Solid Edge part; units mm, degrees
sketch "Sketch1" plane through (0, 0, 0) normal (0, 0, 1) x (1, 0, 0)
  circle A0 centre (0, 0) radius 8.135
extrude "Protrusion1" add sketch "Sketch1" along normal blind 7
sketch "Sketch2" plane through (0, 0, 7) normal (0, 0, 1) x (1, 0, 0)
  line L0 (0, -2.8868) -> (-2.5, -1.4434)
  line L1 (-2.5, -1.4434) -> (-2.5, 1.4434)
  line L2 (-2.5, 1.4434) -> (0, 2.8868)
  line L3 (0, 2.8868) -> (2.5, 1.4434)
  line L4 (2.5, 1.4434) -> (2.5, -1.4434)
  line L5 (2.5, -1.4434) -> (0, -2.8868)
extrude "Cutout1" cut sketch "Sketch2" against normal blind 3.5
sketch "Sketch3" plane through (0, 0, 0) normal (0, 0, -1) x (0, 1, 0)
  circle A0 centre (0, 0) radius 5
extrude "Protrusion2" add sketch "Sketch3" along normal blind 40
sketch "Sketch4" plane through (0, 0, -40) normal (0, 0, -1) x (0, 1, 0)
  circle A0 centre (0, 0) radius 4
extrude "Protrusion3" add sketch "Sketch4" along normal blind 13
chamfer "Chamfer1" distance 0.5 angle 45 1 edges at (0, -4, -53)
properties part number "108082"
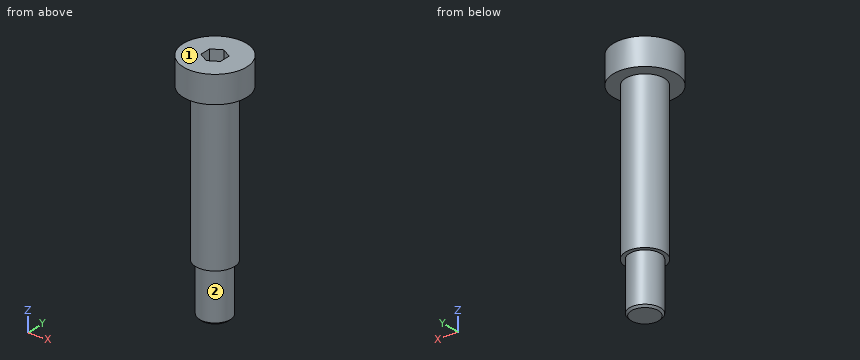
Could you check a few things on this model? Use its own coordinates, in mm. Face numbers are marked on the shaded views. A direction names the side the tool comes from. Round coordinates to 2 decimals unless told otherwise and drop trailing zeros. Loops run counter-clockwise (first coordinate to the right, second up) from the corner with the lowest first, then second, coordinate; pieces in that order, holes last. Notation, with made-up numbers: M 41,43.5 L 55,43.5 A12 cw 55,48.5 Z; hole C -17,27.25 d5. An arc over 180 degrees is marked long. Write item = value, one per line.
1. I want a section at D-D, the plane x = 6. Write out the boundary of the cut face in (y, z), and give its area (3 significant figures).
Results below:
outline = M -5.49,0 L 5.49,0 L 5.49,7 L -5.49,7 Z
area = 76.9 mm²
2. Which directions (+Z, -Z, +X, -X, +Y, -Y) give clear straight access to the entire face, cutting with the end or side of a thin tool? Please do the marked faces 1 and 2.
Results below:
face_1 = +Z, +X, -X, +Y, -Y
face_2 = -Z
3. I want a section at B-B, the plane z = -34. Write out the boundary of the cut face in (x, y).
Results below:
outline = C 0,0 d10
4. Will these pins go through, and if not, where does the flat tip stop? P1, Ø4, axis at x = -4, y = 5.5, coming from the -Z side; P2, Ø6, axis at y = 2.5, z = -8.5, coming from the +X side; P3, Ø1, axis at x = 4.5, z = 0.5, coming from the -Y side.
Results below:
P1 = -40
P2 = 5
P3 = -7.08
5. I need wall thicknesses on probe 1 along Z at (x, y) = (0, 4.25); probe 2 along X at (y, z) = (0, -7); probe 3 along Z at (x, y) = (-1.75, 0.75). Which ranges of each line are inside material? Lowest first, please.
Results below:
probe_1 = -40 to 7
probe_2 = -5 to 5
probe_3 = -53 to 3.5
6. I want a section at C-C, the plane x = -6.75. Write out the boundary of the cut face in (y, z).
Results below:
outline = M -4.54,0 L 4.54,0 L 4.54,7 L -4.54,7 Z
7. I want a section at A-A, the plane y = 0. Write out the boundary of the cut face in (x, z) (3 decimals), and give its area (3 significant figures).
Results below:
outline = M -8.135,0 L -5,0 L -5,-40 L -4,-40 L -4,-52.5 L -3.5,-53 L 3.5,-53 L 4,-52.5 L 4,-40 L 5,-40 L 5,0 L 8.135,0 L 8.135,7 L 2.5,7 L 2.5,3.5 L -2.5,3.5 L -2.5,7 L -8.135,7 Z
area = 600 mm²
